Check sheet for the modelled part. Datum: model origin and axes. Units: mm. Face numbers are marked on the shaded views. A direction names the side the tool comes from. Coordinates: 2 decimals unless noted, no trailing zeros. Loops run counter-clockwise (first coordinate to the right, second up) from the corner with the lowest first, then second, coordinate; pieces in that order, holes last. Notation, with made-up numbers: (80, 73) -> (120, 73) arc R36 cw to (120, 111) -> close; hole circle Ø11 at (54, 66.5). An arc over 180 degrees is marked (long way). Use CSV: the item, a comma, the result in double quotes.
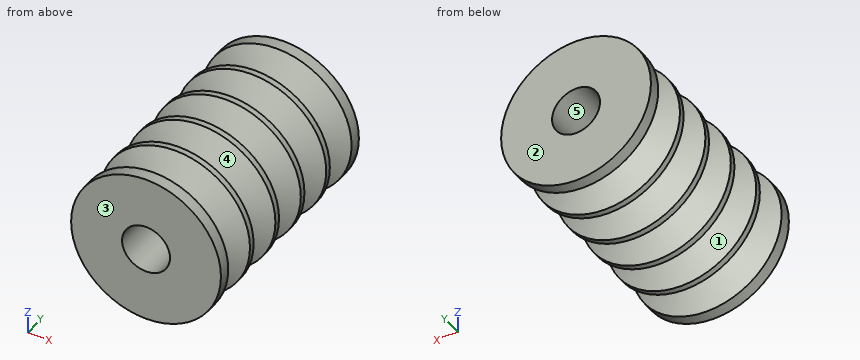
```python
from build123d import *

# Parameters (mm, degrees)
F0_R      = 12.5
F1_DEPTH  = 5
F2_SIZE2  = 6.4335207615
F2_SIZE   = 3
F3_R      = 12.5
F4_DEPTH  = 7
F5_SIZE2  = 6.433511
F5_SIZE   = 2.99999
F6_R      = 12.5
F7_DEPTH  = 7
F8_SIZE2  = 6.433421
F8_SIZE   = 2.9999
F9_R      = 12.5
F10_DEPTH = 7
F11_SIZE2 = 6.432521
F11_SIZE  = 2.999
F12_R     = 12.5
F13_DEPTH = 7
F15_R     = 12.5
F16_DEPTH = 5
F17_SIZE2 = 6.433511
F17_SIZE  = 2.99999
F19_D     = 8


# Not quite as in the source:
# - a fillet or chamfer that OpenCascade refuses, or shapes differently, is made with other operations: its cross-section is extruded or revolved along the edge and cut away or added
# - a fillet or chamfer is up to 0.001 mm smaller than in the source, because OpenCascade refuses the exact size


with BuildPart() as f1:
    # F0 (on Front) → F1 (new body)
    with BuildSketch(Plane.XZ):
        Circle(F0_R)
    extrude(amount=F1_DEPTH)

    # F2
    f2_edges = [f1.edges().sort_by_distance(p)[0] for p in [
        (-12.5, -5, 0),
    ]]
    f2_side = f1.faces().sort_by_distance((-12.5, -2.5, 0))[0]
    chamfer(f2_edges, length=F2_SIZE, length2=F2_SIZE2, reference=f2_side)

    # F3 (on face) → F4 (join)
    with BuildSketch(Plane.XZ.offset(5)):
        Circle(F3_R)
    extrude(amount=F4_DEPTH)

    # F5 (size 3 and 6.4335207615 in the source; OpenCascade refuses exactly that, so slightly less here)
    f5_edges = [f1.edges().sort_by_distance(p)[0] for p in [
        (-12.5, -5, 0),
        (-12.5, -12, 0),
    ]]
    f5_side = f1.faces().sort_by_distance((-12.5, -8.5, 0))[0]
    chamfer(f5_edges, length=F5_SIZE, length2=F5_SIZE2, reference=f5_side)

    # F6 (on face) → F7 (join)
    with BuildSketch(Plane.XZ.offset(12)):
        Circle(F6_R)
    extrude(amount=F7_DEPTH)

    # F8 (size 3 and 6.4335207615 in the source; OpenCascade refuses exactly that, so slightly less here)
    f8_edges = [f1.edges().sort_by_distance(p)[0] for p in [
        (-12.5, -12, 0),
        (-12.5, -19, 0),
    ]]
    f8_side = f1.faces().sort_by_distance((-12.5, -15.5, 0))[0]
    chamfer(f8_edges, length=F8_SIZE, length2=F8_SIZE2, reference=f8_side)

    # F9 (on face) → F10 (join)
    with BuildSketch(Plane.XZ.offset(19)):
        Circle(F9_R)
    extrude(amount=F10_DEPTH)

    # F11 (size 3 and 6.4335207615 in the source; OpenCascade refuses exactly that, so slightly less here)
    f11_edges = [f1.edges().sort_by_distance(p)[0] for p in [
        (-12.5, -19, 0),
        (-12.5, -26, 0),
    ]]
    f11_side = f1.faces().sort_by_distance((-12.5, -22.5, 0))[0]
    chamfer(f11_edges, length=F11_SIZE, length2=F11_SIZE2, reference=f11_side)

    # F12 (on face) → F13 (join)
    with BuildSketch(Plane.XZ.offset(26)):
        Circle(F12_R)
    extrude(amount=F13_DEPTH)

    # F14: chamfer of 3 x 6.4335207615 on 2 edges, made by hand

    # F14_s1 → F14_t2 (revolve, cut)
    with BuildSketch(Plane.XY):
        Polygon((12.5, -29), (6.0664792385, -26), (12.5, -26), align=None)
    revolve(axis=Axis((0, -26, 0), (0, -1, 0)), mode=Mode.SUBTRACT)

    # F14_s3 → F14_t4 (revolve, cut)
    with BuildSketch(Plane.XY):
        Polygon((12.5, -30), (6.0664792385, -33), (12.5, -33), align=None)
    revolve(axis=Axis((0, -33, 0), (0, -1, 0)), mode=Mode.SUBTRACT)

    # F15 (on face) → F16 (join)
    with BuildSketch(Plane.XZ.offset(33)):
        Circle(F15_R)
    extrude(amount=F16_DEPTH)

    # F17 (size 3 and 6.4335207615 in the source; OpenCascade refuses exactly that, so slightly less here)
    f17_edges = [f1.edges().sort_by_distance(p)[0] for p in [
        (-12.5, -33, 0),
    ]]
    f17_side = f1.faces().sort_by_distance((-12.5, -35.5, 0))[0]
    chamfer(f17_edges, length=F17_SIZE, length2=F17_SIZE2, reference=f17_side)

    # F19 (through all)
    with Locations(Plane(origin=(0, 0, 0), x_dir=(-1, 0, 0), z_dir=(0, 1, 0))):
        with Locations((0, 0)):
            Hole(F19_D / 2)


solid = f1.part
```
1) Cross-section at A-A on z = 8.75. Give the number of separate pieces and of enclosed holes in the cut face, and give its area (3 significant figures).
Answer below:
separate pieces,"6"
enclosed holes,"0"
area,"343 mm²"
2) Go/stop test with flat-tipped pins: pin 1 Ø10 at (y, z) = (-30, -6) entering from -X; pin 2 Ø5 at (x, z) = (0, 0) entering from -Y. Record where each tip stops, or that it passes through.
Answer below:
pin 1,"stops at x = -12.46"
pin 2,"passes through"
3) Draft check along Y on the marked faces 1, 2 and 3. Enter one of: released by +Y, released by -Y, zero draft, split by the parting line, or undercut.
Answer below:
face 1,"undercut"
face 2,"released by +Y"
face 3,"released by -Y"
4) Cross-section at D-D on y = -32. Record the boundary of the cut face in (x, z), and give its area (3 significant figures).
Answer below:
outline,"circle Ø16.42 at (0, 0); hole circle Ø8 at (0, 0)"
area,"162 mm²"
5) Access from +Z, -Z, +X, -X, +Y, -Y to the whole of each face (thin tool, end or side, straight path). Record for the marked faces 4 and 5.
Answer below:
face 4,"none"
face 5,"+Y, -Y"
6) Thickness scan on line 1 along Y through (x, z) = (-10, 2.25); line 2 along Y through (x, z) = (-10.5, -5.75); line 3 along Z through (x, y) = (0, -21). Record the ranges inside material, lowest first. Write a range as from..to.
Answer below:
line 1,"y = -38..-34.95, -31.05..-27.95, -24.05..-20.95, -17.05..-13.95, -10.05..-6.95, -3.05..0"
line 2,"y = -38..-35.75, -30.25..-28.75, -23.25..-21.75, -16.25..-14.75, -9.25..-7.75, -2.25..0"
line 3,"z = -10.36..-4, 4..10.36"
7) Cross-section at C-C on y = -26.5. Record the boundary of the cut face in (x, z), and give its area (3 significant figures).
Answer below:
outline,"circle Ø14.28 at (0, 0); hole circle Ø8 at (0, 0)"
area,"110 mm²"
